Geometry check sheet. Reference: the model listing, model coordinates, mm. Face numbers are marked on the shaded views. A direction names the side the tool comes from. Give positions to 0.01 mm unless a question says otherwise; leave off trailing zeros. Loops run counter-clockwise (first coordinate to the right, second up) from the corner with the lowest first, then second, coordinate; pieces in that order, holes last. Notation, with made-up numbers: (-14, 53.25) - (13, 53.25) arc R28 ccw to (13, 85.25) - close; hole circle Ø9 at (-12, 35.25). An arc over 180 degrees is marked (long way). Use a Markdown table: item, result. Add a question column.
1. Depth check by flat-ended pin: P1, Ø3.5, axis at x = 25, y = 0, coming from the -Z side; P2, Ø2.5, axis at y = 15.01, z = 41, coming from the +X side; P3, Ø2.5, axis at y = -14.58, z = 23.9, coming from the -X side; P4, Ø4, axis at y = -14.58, z = 15.9, coming from the -X side. Enter the tip coordinate at first touch or a pass-through.
2. Draft check along Y on the marked faces 1, 2 and 3. Enter one of: pulls with the +Y half, pulls with the -Y half, needs draft (parallel to the pull), parting line crosses it, or undercut.
3. Cross-section at A-A on y = -25. Enter the section's corners in (x, z), and give its area (4 significant figures).
4. Cross-section at D-D on y = 25. Enter the section's corners in (x, z), and give its area (3 significant figures).
5. Cross-section at B-B on x = 25. Enter the section's corners in (y, z).
6. Cross-section at C-C on x = 0. Enter the section's corners in (y, z), and give its area (3 significant figures).
7. Set-up check for the marked faces 4, 5 and 6: record each of +Z, -Z, +X, -X, +Y, -Y from which the full face is reachable in a straight line by a thin tool's end or side.
8. Material ranges on L1, parallel to Y at x = -31, z = 41; L2, parallel to Y at x = -42.25, z = 19.9; L3, parallel to Y at x = 25, z = 1.7, recorded low to high.
Autodesk Inventor part; units mm, degrees
ref_plane "Work Plane2" through (-93.15, -42.6288, 31.9788) normal (0, 0, -1) x (0, 1, 0)
ref_plane "YZ Plane" through (0, 0, 0) normal (1, 0, 0) x (0, 1, 0)
ref_plane "XZ Plane" through (0, 0, 0) normal (0, 1, 0) x (-1, 0, 0)
ref_plane "Work Plane1" through (0, 0, 0) normal (0, 0, 1) x (1, 0, 0)
sketch "Sketch1" plane through (0, 0, 0) normal (0, 0, 1) x (1, 0, 0)
  circle A0 centre (25, 25) radius 1.95
  circle A1 centre (25, 0) radius 1.95
  circle A2 centre (0, 25) radius 1.95
  circle A3 centre (-25, 0) radius 1.95
  circle A4 centre (-25, -25) radius 1.95
  circle A5 centre (25, 25) radius 1.95
  circle A6 centre (25, -25) radius 1.95
  circle A7 centre (-25, 25) radius 1.95
  circle A8 centre (25, 0) radius 1.95
  circle A9 centre (0, -25) radius 1.95
  line L0 (-28, 30) -> (-30, 28)
  line L1 (-30, 28) -> (-30, -28)
  line L2 (-30, -28) -> (-28, -30)
  line L3 (-28, -30) -> (28, -30)
  line L4 (28, -30) -> (30, -28)
  line L5 (30, -28) -> (30, 28)
  line L6 (30, 28) -> (28, 30)
  line L7 (28, 30) -> (-28, 30)
  point P0 (0, 0)
extrude "Extrusion1" add sketch "Sketch1" along normal blind 5
sketch "Sketch2" plane through (0, 0, 5) normal (0, 0, 1) x (1, 0, 0)
  circle A0 centre (0, -25) radius 1.95
  circle A1 centre (-25, 25) radius 1.95
  circle A2 centre (25, -25) radius 1.95
  circle A3 centre (-25, -25) radius 1.95
  circle A4 centre (-25, 0) radius 1.95
  circle A5 centre (0, 25) radius 1.95
  circle A6 centre (25, 0) radius 1.95
  circle A7 centre (25, 25) radius 1.95
  line L0 (-28, 30) -> (-30, 28)
  line L1 (-30, 28) -> (-30, -28)
  line L2 (-30, -28) -> (-28, -30)
  line L3 (-28, -30) -> (28, -30)
  line L4 (28, -30) -> (30, -28)
  line L5 (30, -28) -> (30, 28)
  line L6 (30, 28) -> (28, 30)
  line L7 (28, 30) -> (-28, 30)
  line L8 (-30, 28) -> (-30, -28)
  line L9 (-30, -22) -> (22, -22)
  line L10 (22, -22) -> (22, 22)
  line L11 (22, 22) -> (-30, 22)
  line L12 (-30, 22) -> (-30, -22)
  point P0 (0, 0)
  dimension "d2" = 8
  dimension "d3" = 8
  dimension "d4" = 8
ref_plane "Work Plane2" through (-93.15, -42.6288, 31.9788) normal (0, 0, -1) x (0, 1, 0)
extrude "Extrusion2" add sketch "Sketch2" along normal blind 40 contours A4 | L11 L10 L9 L1
sketch "Sketch3" plane through (-30, -28, 0) normal (-1, 0, 0) x (0, 0, 1)
  line L0 (0, 56) -> (0, 0)
  line L1 (0, 0) -> (5, 0)
  line L2 (5, 6) -> (5, 0)
  line L3 (5, 6) -> (45, 6)
  line L4 (5, 50) -> (45, 50)
  line L5 (5, 56) -> (5, 50)
  line L6 (0, 56) -> (5, 56)
  line L7 (45, 50) -> (45, 6)
  point P0 (0, 28)
extrude "Extrusion3" add sketch "Sketch3" along normal blind 10
sketch "Sketch4" plane through (22, -22, 0) normal (0, 0, 1) x (1, 0, 0)
  line L0 (-62, 0) -> (0, 0)
  line L1 (0, 44) -> (-62, 44)
  line L2 (-62, 0) -> (-62, 44)
  arc A0 (-111.65, 45.2512) -> (-115.15, 41.7512) centre (-111.65, 41.7512) ccw
  line L3 (-115.15, -17.1288) -> (-115.15, 41.7512)
  arc A1 (-115.15, -17.1288) -> (-111.65, -20.6288) centre (-111.65, -17.1288) ccw
  line L4 (28.35, -20.6288) -> (-111.65, -20.6288)
  arc A2 (28.35, -20.6288) -> (31.85, -17.1288) centre (28.35, -17.1288) ccw
  line L5 (31.85, 41.7512) -> (31.85, -17.1288)
  arc A3 (31.85, 41.7512) -> (28.35, 45.2512) centre (28.35, 41.7512) ccw
  line L6 (-111.65, 45.2512) -> (28.35, 45.2512)
  line L7 (0, 0) -> (0, 44)
  line L8 (-62, 44) -> (0, 44)
  line L9 (0, 44) -> (0, 0)
  line L10 (0, 0) -> (-62, 0)
  line L11 (-62, 0) -> (-62, 44)
  line L12 (-5, 39) -> (-57, 39)
  line L13 (-57, 39) -> (-57, 5)
  line L14 (-57, 5) -> (-5, 5)
  line L15 (-5, 5) -> (-5, 39)
  point P0 (-22, 22)
  dimension "d9" = 5
extrude "Extrusion4" cut sketch "Sketch4" along normal blind 40 contours L15 L14 L13 L12
sketch "Sketch6" plane through (-40, -28, 0) normal (-1, 0, 0) x (0, 0, 1)
  line L0 (0, 56) -> (0, 0)
  line L1 (0, 0) -> (5, 0)
  line L2 (5, 0) -> (5, 6)
  line L3 (5, 6) -> (45, 6)
  line L4 (45, 50) -> (5, 50)
  line L5 (5, 50) -> (5, 56)
  line L6 (5, 56) -> (0, 56)
  line L7 (45, 6) -> (45, 50)
  point P0 (0, 28)
extrude "Extrusion6" add sketch "Sketch6" along normal blind 5
sketch "Sketch7" plane through (-45, -28, 0) normal (-1, 0, 0) x (0, 0, 1)
  circle A0 centre (41, 25.7717) radius 1.45
  circle A1 centre (23.9, 21.2512) radius 1.45
  circle A2 centre (3.3174, 32.2512) radius 1.45
  circle A3 centre (3.3174, 53) radius 1.45
  line L0 (40, 45) -> (40, 11)
  circle A4 centre (41, 8.1883) radius 1.45
  circle A5 centre (4.9143, 21.2512) radius 1.45
  circle A6 centre (23.9337, 3.5995) radius 1.45
  circle A7 centre (41, 25.7717) radius 1.45
  circle A8 centre (41.0502, 56) radius 1.45
  circle A9 centre (41, 0.7395) radius 1.45
  circle A10 centre (23.9, 21.2512) radius 1.45
  circle A11 centre (23.9, 13.4229) radius 1.45
  circle A12 centre (41, 43.0063) radius 1.45
  line L1 (37.1004, -11.7636) -> (45, -11.7636)
  line L2 (45, -11.7636) -> (45, 58)
  line L3 (26.9, 58) -> (26.9, 25.2512)
  line L4 (26.9, 25.2512) -> (-10.2763, 25.2512)
  line L5 (-10.2763, 25.2512) -> (37.1004, -11.7636)
  line L6 (45, 58) -> (26.9, 58)
  point P0 (0, 28)
  point P1 (4.6577, 21.4172)
hole "Hole1" at (-45, 15.0063, 41) at (-45, -2.2283, 41) at (-45, -19.8117, 41) at (-45, -14.5771, 23.9) at (-45, -6.7488, 23.9) at (-45, 4.2512, 3.3174) at (-45, 25, 3.3174) at (-45, -6.7488, 4.9143) direction (1, 0, 0) diameter 2.9 depth 20 tip angle 118
pattern_linear "Rectangular Pattern1" count 4 spacing 4 along (0, 0, -1) of "Hole1"
properties part number "cellSTORM_v5_cellphonestage"
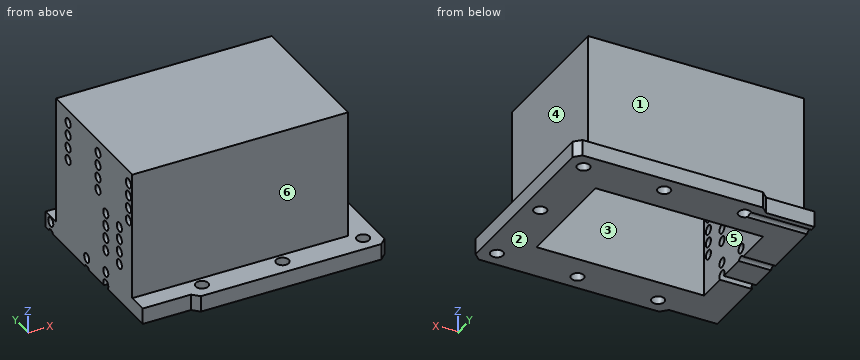
Values found:
| question | item | result |
|---|---|---|
| 1 | P1 | passes through |
| 1 | P2 | stops at x = 22 |
| 1 | P3 | stops at x = 17 |
| 1 | P4 | stops at x = -45 |
| 2 | face 1 | pulls with the +Y half |
| 2 | face 2 | needs draft |
| 2 | face 3 | undercut |
| 3 | outline | (-45, 0) - (-26.95, 0) - (-26.95, 5) - (-45, 5) - close; (-23.05, 0) - (-1.95, 0) - (-1.95, 5) - (-23.05, 5) - close; (1.95, 0) - (23.05, 0) - (23.05, 5) - (1.95, 5) - close; (26.95, 0) - (30, 0) - (30, 5) - (26.95, 5) - close |
| 3 | area | 316.5 mm2 |
| 4 | outline | (-45, 0.77) - (-26.95, 0.77) - (-26.95, 1.87) - (-45, 1.87) - close; (-45, 4.77) - (-26.95, 4.77) - (-26.95, 5) - (-45, 5) - close; (-23.05, 0) - (-1.95, 0) - (-1.95, 5) - (-23.05, 5) - close; (1.95, 0) - (23.05, 0) - (23.05, 5) - (1.95, 5) - close; (26.95, 0) - (30, 0) - (30, 5) - (26.95, 5) - close |
| 4 | area | 250 mm2 |
| 5 | outline | (-30, 0) - (-26.95, 0) - (-26.95, 5) - (-30, 5) - close; (-23.05, 0) - (-1.95, 0) - (-1.95, 5) - (-23.05, 5) - close; (1.95, 0) - (23.05, 0) - (23.05, 5) - (1.95, 5) - close; (26.95, 0) - (30, 0) - (30, 5) - (26.95, 5) - close |
| 6 | outline | (-30, 0) - (-26.95, 0) - (-26.95, 5) - (-30, 5) - close; (-23.05, 0) - (-17, 0) - (-17, 40) - (17, 40) - (17, 0) - (23.05, 0) - (23.05, 5) - (22, 5) - (22, 45) - (-22, 45) - (-22, 5) - (-23.05, 5) - close; (26.95, 0) - (30, 0) - (30, 5) - (26.95, 5) - close |
| 6 | area | 661 mm2 |
| 7 | face 4 | +Z, +X, +Y, -Y |
| 7 | face 5 | -Z |
| 7 | face 6 | +Z, +X, -X, -Y |
| 8 | L1 | y = -22 to -21.26, -18.36 to -3.68, -0.78 to 13.56, 16.46 to 22 |
| 8 | L2 | y = -22 to -16.03, -13.13 to -8.2, -5.3 to 22 |
| 8 | L3 | y = -30 to -26.95, -23.05 to -1.95, 1.95 to 23.05, 26.95 to 30 |
